Geometry: see drawing. Coordinates: mm, zero at the bounding-box minimum. A direction names the side the tool comes from. Coordinates: 2 decimals unless noted, no trailing zeros. Order: outer loops, then holes, each group sorted by start corner. A loop starts at its lowest first (then second) coordinate and runs counter-clockwise, first axis right, second up. Notation, with made-up numbers: (74, -19.5) -> (116, -19.5) arc R21 cw to (116, -1.5) -> close; hole circle Ø10 at (-15, -24). An arc over 180 degrees is marked (long way). Use one line per item in the form item = value.
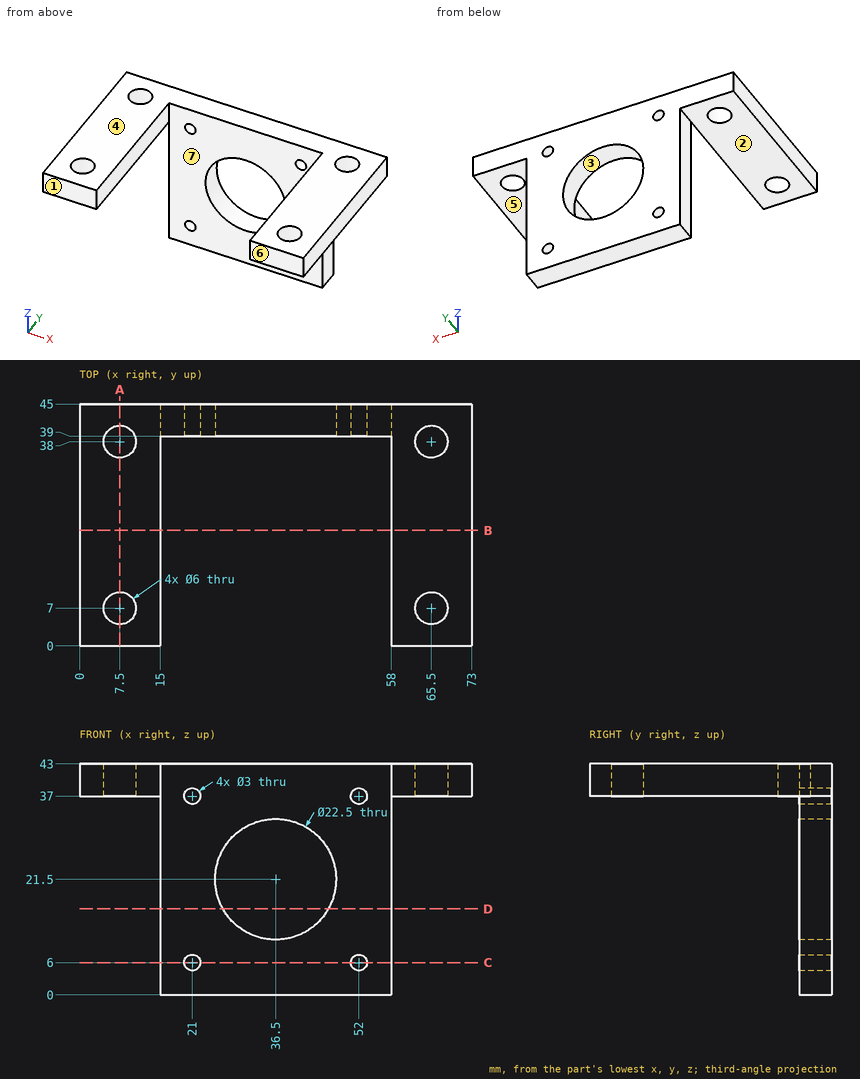
1) Section A-A, the plane x = 7.5. Output: boundary loops of the cut face in (y, z).
Results found:
outline = (0, 37) -> (4, 37) -> (4, 43) -> (0, 43) -> close; (10, 37) -> (35, 37) -> (35, 43) -> (10, 43) -> close; (41, 37) -> (45, 37) -> (45, 43) -> (41, 43) -> close
2) Section D-D, the plane z = 16. Output: boundary loops of the cut face in (x, y).
Results found:
outline = (15, 39) -> (26.69, 39) -> (26.69, 45) -> (15, 45) -> close; (46.31, 39) -> (58, 39) -> (58, 45) -> (46.31, 45) -> close
3) Material intervals for probe 1 along X at (y, z) = (43.3, 6); probe 2 along X at (y, z) = (42.25, 21.5); probe 3 along Y at (x, z) = (7, 39), sorted ascending. Write a range as from..to.
Results found:
probe_1 = 15..19.5, 22.5..50.5, 53.5..58
probe_2 = 15..25.25, 47.75..58
probe_3 = 0..4.04, 9.96..35.04, 40.96..45
4) Contact query for flat-ended pins moving along their axis: P1, Ø20, axis at x = 36.5, z = 21.5, coming from the +Y side; P2, Ø16.5, axis at x = 67.5, y = 11.5, coming from the -Z side; P3, Ø5, axis at x = 52, z = 6, coming from the -Y side; P4, Ø5, axis at y = 41.5, z = 24.5, coming from the -X side. Output: stop coordinate, or through.
Results found:
P1 = through
P2 = 37
P3 = 39
P4 = 15
5) Section B-B, the plane y = 21.5. Output: boundary loops of the cut face in (x, z).
Results found:
outline = (0, 37) -> (15, 37) -> (15, 43) -> (0, 43) -> close; (58, 37) -> (73, 37) -> (73, 43) -> (58, 43) -> close
6) Section C-C, the plane z = 6. Output: boundary loops of the cut face in (x, y), and give its area (3 significant figures).
Results found:
outline = (15, 39) -> (19.5, 39) -> (19.5, 45) -> (15, 45) -> close; (22.5, 39) -> (50.5, 39) -> (50.5, 45) -> (22.5, 45) -> close; (53.5, 39) -> (58, 39) -> (58, 45) -> (53.5, 45) -> close
area = 222 mm2
7) Pull-direction query (Z, two-part tool) for the marked faces 1, 2, 3 and 4; classes: released by +Z, released by -Z, zero draft, split by the parting line, or undercut.
Results found:
face_1 = zero draft
face_2 = released by -Z
face_3 = undercut
face_4 = released by +Z
8) Access query for the marked faces 5, 6 and 7. Directions: +Z, -Z, +X, -X, +Y, -Y. A direction counts if a zero-diameter tool reaches every point of the face in a straight line with its end or side. Return the directions, or none.
Results found:
face_5 = -Z, +X, +Y, -Y
face_6 = +Z, -Z, +X, -X, -Y
face_7 = +Z, -Z, -Y
